Source: three-view drawing plus pictorial views. Frame: mm from the lowest corner of the part. Coordinates: 2 decimals unless noted, no trailing zeros. Loops run counter-clockwise (first coordinate to the right, second up) from the corner with the lowest first, then second, coordinate; pieces in that order, holes last. Notation, with made-up numbers: (8.5, -12) -> (65.5, -12) arc R19 cw to (65.5, -4) -> close; hole circle Ø3 at (30, -21). An arc over 180 degrees is marked (long way). Answer as a JSON object with one key per item and string values. Group by question number.
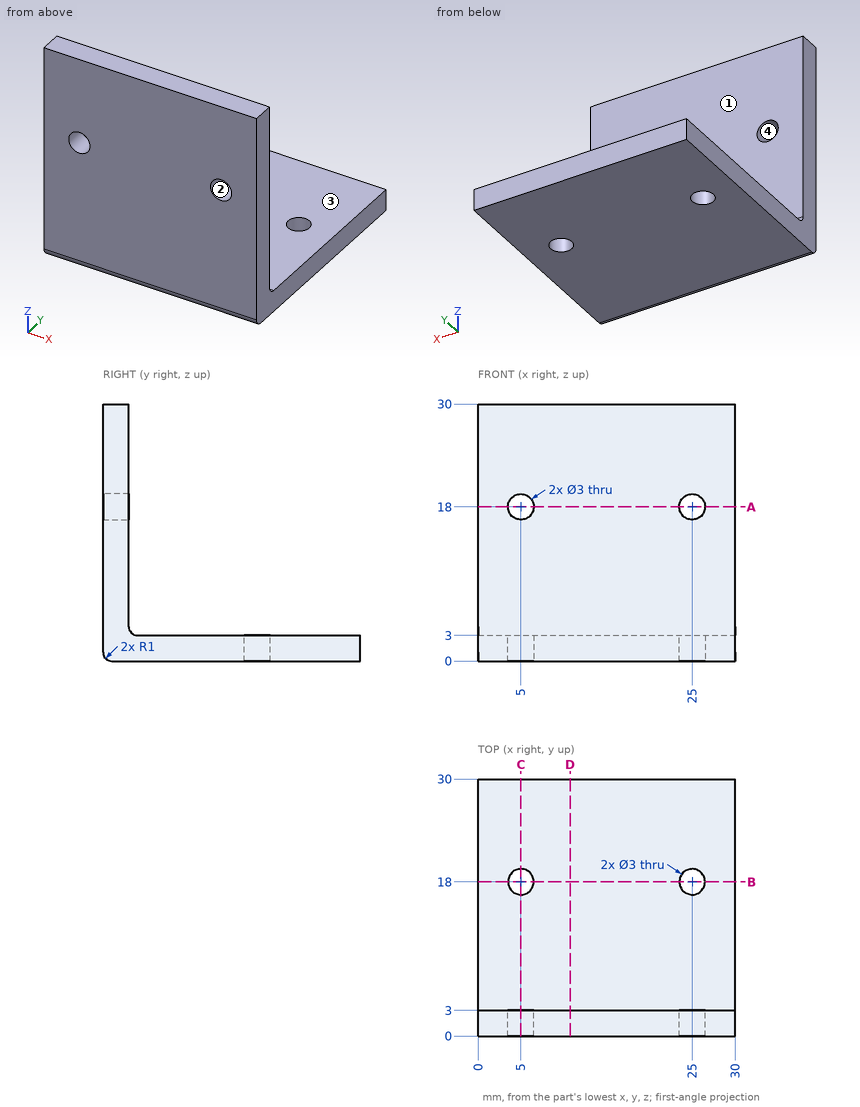
1. Section query A-A on z = 18. Return loops of the section in (x, y).
2. Section query C-C on x = 5. Return loops of the section in (y, z).
3. Mould query, pull axis Z, two halves, no side actions, for the marked faces 1, 2, 3 and 4. Classes: pulls with the +Z half, pulls with the -Z half, needs draft (parallel to the pull), parting line crosses it, or undercut.
4. Section query D-D on x = 10.75. Return loops of the section in (y, z).
5. Ray query, L1, parallel to X at y = 1.05, z = 18; L2, parallel to Y at x = 25, z = 0.9; L3, parallel to Z at x = 24.75, y = 7. Return the intervals inside material, ascending.
6. Pin query (flat end, axial travel): pin 1 Ø10 at (x, z) = (12.5, 9) entering from -Y; pin 2 Ø6 at (x, y) = (21.5, 9.5) entering from +Z; pin 3 Ø2.5 at (x, z) = (25, 18) entering from +Y. Return the tip coordinate at first contact, or that it passes through.
Solved:
{
 "1": {"outline": "(0, 0) -> (3.5, 0) -> (3.5, 3) -> (0, 3) -> close; (6.5, 0) -> (23.5, 0) -> (23.5, 3) -> (6.5, 3) -> close; (26.5, 0) -> (30, 0) -> (30, 3) -> (26.5, 3) -> close"},
 "2": {"outline": "(0, 1) arc R1 ccw to (1, 0) -> (16.5, 0) -> (16.5, 3) -> (4, 3) arc R1 cw to (3, 4) -> (3, 16.5) -> (0, 16.5) -> close; (0, 19.5) -> (3, 19.5) -> (3, 30) -> (0, 30) -> close; (19.5, 0) -> (30, 0) -> (30, 3) -> (19.5, 3) -> close"},
 "3": {"face 1": "needs draft", "face 2": "undercut", "face 3": "pulls with the +Z half", "face 4": "undercut"},
 "4": {"outline": "(0, 1) arc R1 ccw to (1, 0) -> (30, 0) -> (30, 3) -> (4, 3) arc R1 cw to (3, 4) -> (3, 30) -> (0, 30) -> close"},
 "5": {"L1": "0 to 3.5, 6.5 to 23.5, 26.5 to 30", "L2": "0.01 to 16.5, 19.5 to 30", "L3": "0 to 3"},
 "6": {"pin 1": "y = 0", "pin 2": "z = 3", "pin 3": "through"}
}
